Build history of the part. All positions in model axes, mm. Face numbers are marked on the shaded views. A direction names the side the tool comes from. Round coordinates to 2 decimals unless told otherwise and drop trailing zeros. Order: outer loops, then holes, each group sorted by start corner. A loop starts at its lowest first (then second) coordinate and runs counter-clockwise, first axis right, second up. Notation, with made-up numbers: M 22.25,9.5 L 75.25,9.5 A21 cw 75.25,33.5 Z; hole C 57,16.5 d6. An arc over 180 degrees is marked long. Use CSV: the item, a comma, the result in double quotes.
from build123d import *

# Parameters (mm, degrees)
SKETCH1_W           = 100
SKETCH1_H           = 60
SKETCH1_R           = 2
SKETCH1_W_2         = 80
SKETCH1_H_2         = 20
BOSS_EXTRUDE1_DEPTH = 10


with BuildPart() as part:
    # Sketch1 → Boss-Extrude1 (new body)
    with BuildSketch(Plane(origin=(0, 0, 0), x_dir=(1, 0, 0), z_dir=(0, 1, 0))):
        with Locations((50, 30)):
            Rectangle(SKETCH1_W, SKETCH1_H)
        with Locations(Location((5, 30, 0), (0, 0, 270))):
            Circle(SKETCH1_R, mode=Mode.SUBTRACT)
        with Locations(Location((5, 50, 0), (0, 0, 270))):
            Circle(SKETCH1_R, mode=Mode.SUBTRACT)
        with Locations(Location((5, 10, 0), (0, 0, 270))):
            Circle(SKETCH1_R, mode=Mode.SUBTRACT)
        with Locations(Location((15, 50, 0), (0, 0, 270))):
            Circle(SKETCH1_R, mode=Mode.SUBTRACT)
        with Locations(Location((15, 10, 0), (0, 0, 270))):
            Circle(SKETCH1_R, mode=Mode.SUBTRACT)
        with Locations(Location((25, 50, 0), (0, 0, 270))):
            Circle(SKETCH1_R, mode=Mode.SUBTRACT)
        with Locations(Location((25, 10, 0), (0, 0, 270))):
            Circle(SKETCH1_R, mode=Mode.SUBTRACT)
        with Locations(Location((35, 50, 0), (0, 0, 270))):
            Circle(SKETCH1_R, mode=Mode.SUBTRACT)
        with Locations(Location((35, 10, 0), (0, 0, 270))):
            Circle(SKETCH1_R, mode=Mode.SUBTRACT)
        with Locations(Location((45, 50, 0), (0, 0, 270))):
            Circle(SKETCH1_R, mode=Mode.SUBTRACT)
        with Locations(Location((45, 10, 0), (0, 0, 270))):
            Circle(SKETCH1_R, mode=Mode.SUBTRACT)
        with Locations(Location((55, 50, 0), (0, 0, 270))):
            Circle(SKETCH1_R, mode=Mode.SUBTRACT)
        with Locations(Location((55, 10, 0), (0, 0, 270))):
            Circle(SKETCH1_R, mode=Mode.SUBTRACT)
        with Locations(Location((65, 50, 0), (0, 0, 270))):
            Circle(SKETCH1_R, mode=Mode.SUBTRACT)
        with Locations(Location((65, 10, 0), (0, 0, 270))):
            Circle(SKETCH1_R, mode=Mode.SUBTRACT)
        with Locations(Location((75, 50, 0), (0, 0, 270))):
            Circle(SKETCH1_R, mode=Mode.SUBTRACT)
        with Locations(Location((75, 10, 0), (0, 0, 270))):
            Circle(SKETCH1_R, mode=Mode.SUBTRACT)
        with Locations(Location((85, 50, 0), (0, 0, 270))):
            Circle(SKETCH1_R, mode=Mode.SUBTRACT)
        with Locations(Location((85, 10, 0), (0, 0, 270))):
            Circle(SKETCH1_R, mode=Mode.SUBTRACT)
        with Locations(Location((95, 50, 0), (0, 0, 270))):
            Circle(SKETCH1_R, mode=Mode.SUBTRACT)
        with Locations(Location((95, 10, 0), (0, 0, 270))):
            Circle(SKETCH1_R, mode=Mode.SUBTRACT)
        with Locations(Location((95, 30, 0), (0, 0, 270))):
            Circle(SKETCH1_R, mode=Mode.SUBTRACT)
        with Locations((50, 30)):
            Rectangle(SKETCH1_W_2, SKETCH1_H_2, mode=Mode.SUBTRACT)
    extrude(amount=BOSS_EXTRUDE1_DEPTH)


solid = part.part
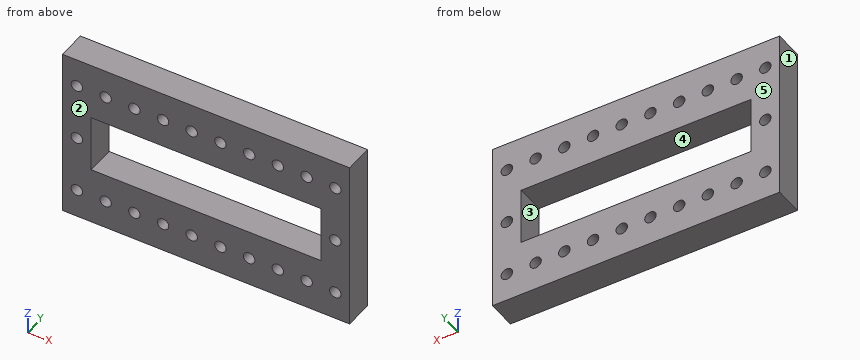
(1) Cut at B-B, the plane z = -33. Give the cut face in (x, y).
Answer block:
outline,"M 0,0 L 10,0 L 10,10 L 0,10 Z; M 90,0 L 100,0 L 100,10 L 90,10 Z"
(2) Cut at D-D, the plane y = 1.75. Count the separate pieces of the cut face and the enclosed holes in it, and give its area (3 significant figures).
Answer block:
separate pieces,"1"
enclosed holes,"23"
area,"4,120 mm²"
(3) Two-plate mould, pull along X, no slides. Class the marked faces 1, 2 and 3: released by +X, released by -X, zero draft, split by the parting line, or undercut.
Answer block:
face 1,"released by -X"
face 2,"zero draft"
face 3,"undercut"
(4) Cut at C-C, the plane x = 69. Give the cut face in (y, z), and give its area (3 significant figures).
Answer block:
outline,"M 0,-60 L 10,-60 L 10,-40 L 0,-40 Z; M 0,-20 L 10,-20 L 10,0 L 0,0 Z"
area,"400 mm²"
(5) Cut at A-A, the plane x = 15. Give the cut face in (y, z), and give its area (3 significant figures).
Answer block:
outline,"M 0,-60 L 10,-60 L 10,-52 L 0,-52 Z; M 0,-48 L 10,-48 L 10,-40 L 0,-40 Z; M 0,-20 L 10,-20 L 10,-12 L 0,-12 Z; M 0,-8 L 10,-8 L 10,0 L 0,0 Z"
area,"320 mm²"
(6) Wall check: line 1 (X direction, y = 5.5, z = -37); line 2 (Z direction, x = 18, y = 8); line 3 (Z direction, x = 84, y = 2.25). Give the ranges that are in metal, low to high. Write a range as from..to.
Answer block:
line 1,"x = 0..10, 90..100"
line 2,"z = -60..-40, -20..0"
line 3,"z = -60..-51.73, -48.27..-40, -20..-11.73, -8.27..0"
(7) Drop a flat-ended pin along its axis: pin 1 (3 mm diameter, centred on x = 85, z = -10, fed in from -Y). Give the stop position or say it passes through.
Answer block:
pin 1,"passes through"
(8) Tool access for the marked faces 4 and 5: list every direction of +Z, -Z, +X, -X, +Y, -Y with a clear straight run to the whole face (end or side of a thin tool).
Answer block:
face 4,"+Y, -Y"
face 5,"+Z, -Z, +X, -X, +Y"
